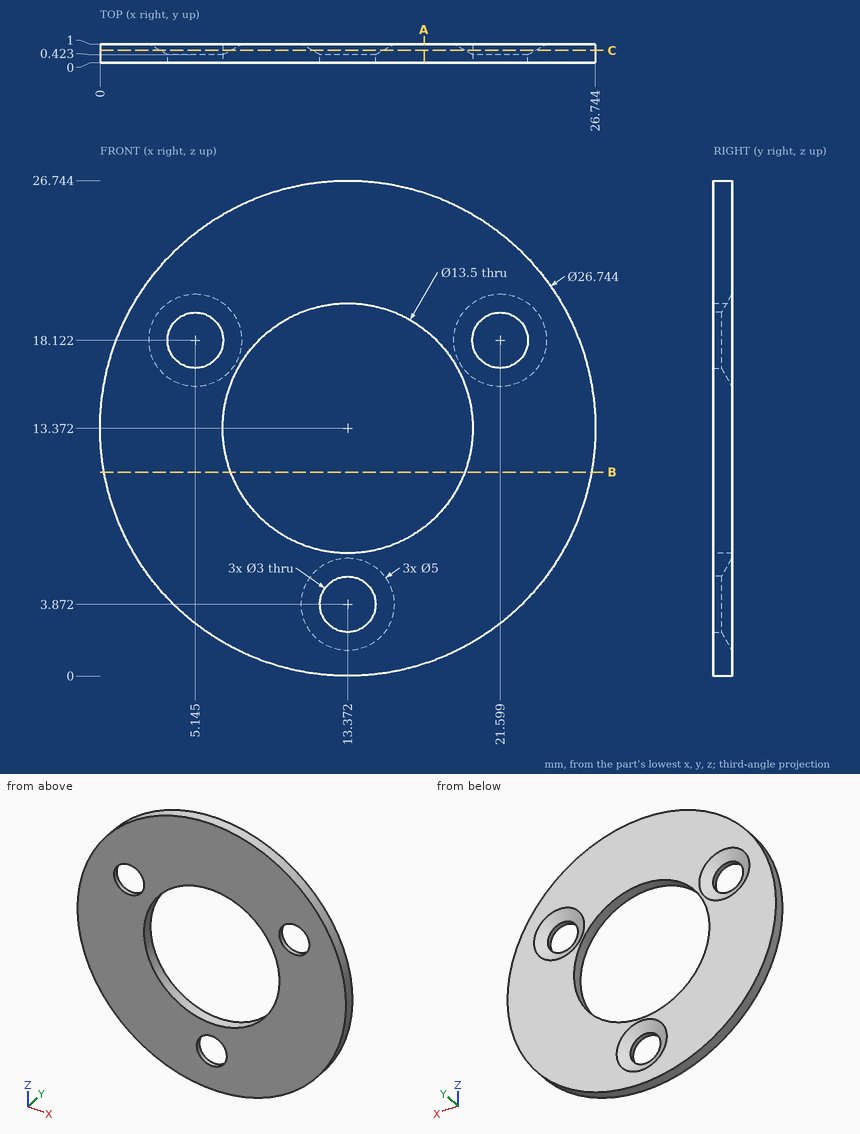
Verification items for this drawing (mm, ordinates from the low corner). Round coordinates to 2 decimals unless told otherwise and drop trailing zeros. Loops run counter-clockwise (first coordinate to the right, second up) from the corner with the lowest first, then second, coordinate; pieces in that order, holes last. Notation, with made-up numbers: (42, 11.5) -> (60, 11.5) arc R24 ccw to (60, 29.5) -> close; hole circle Ø7 at (45, 18.25). An arc over 180 degrees is marked (long way). Write item = value, one per line. Start each with the question number.
1) Sectioned sample at B-B, the plane z = 11. Record the cut outline in (x, y).
2) Sectioned sample at A-A, the plane x = 17.5. Record the cut outline in (y, z).
3) Sectioned sample at C-C, the plane y = 0.65. State how many separate pieces and enclosed holes the cut face has, plus the area to 3 significant figures.
4) Thickness scan on probe 1 along Z at (x, y) = (12, 0.4) (1 decimal); probe 2 along X at (y, z) = (0.15, 17.25) (1 decimal); probe 3 along X at (y, z) = (0.5, 4.5) (1 decimal). Record the ranges inside material, lowest first.
5) Gauge pin test, flat end, axial feed: pin 1 Ø8 at (x, z) = (13.37, 13.37) entering from -Y. Record the tip position at first contact, or that the pin passes through.
Results are:
q1.outline = (0.21, 0) -> (7.05, 0) -> (7.05, 1) -> (0.21, 1) -> close; (19.69, 0) -> (26.53, 0) -> (26.53, 1) -> (19.69, 1) -> close
q2.outline = (0, 0.65) -> (1, 0.65) -> (1, 8.03) -> (0, 8.03) -> close; (0, 18.71) -> (1, 18.71) -> (1, 26.09) -> (0, 26.09) -> close
q3.separate_pieces = 1
q3.enclosed_holes = 4
q3.area = 385 mm^2
q4.probe_1 = 0.1 to 3.3, 4.5 to 6.8, 20 to 26.7
q4.probe_2 = 0.6 to 3.9, 6.4 to 7.8, 18.9 to 20.4, 22.8 to 26.2
q4.probe_3 = 3.4 to 11.9, 14.9 to 23.4
q5.pin_1 = through
